Can you work these out from the model? Positions are in its coordinate system, mm. Face numbers are marked on the shaded views. A direction names the side the tool comes from. Coordinates: 2 decimals unless noted, no trailing zeros. Order: outer loops, then holes, each group sorted by start corner. A loop starts at its lowest first (then second) coordinate and runs counter-clockwise, first axis right, second up.
```python
from build123d import *

# Parameters (mm, degrees)
SKETCH1_W           = 3
SKETCH1_H           = 8.5
BOSS_EXTRUDE1_DEPTH = 0.25
SKETCH4_W           = 3
SKETCH4_H           = 0.5
CUT_EXTRUDE1_DEPTH  = 10.548715932
CHAMFER1_SIZE       = 0.7


with BuildPart() as part:
    # Sketch1 → Boss-Extrude1 (new body, symmetric)
    with BuildSketch(Plane(origin=(0, 0, 0), x_dir=(1, 0, 0), z_dir=(0, 1, 0))):
        Rectangle(SKETCH1_W, SKETCH1_H)
    extrude(amount=BOSS_EXTRUDE1_DEPTH, both=True)

    # Sweep1: sweep along a path in Sketch5
    with BuildLine(Plane(origin=(0, 0, 0), x_dir=(0, 0, -1), z_dir=(1, 0, 0))) as sweep1_path:
        Line((-6.415063509, -3.25), (-4.683012702, -0.25))
        ThreePointArc((-4.683012702, -0.25), (-4.5, -0.066987298), (-4.25, 0))
    # Sketch4 → Sweep1 (sweep)
    with BuildSketch(Plane.XY.offset(4.25)):
        Rectangle(SKETCH4_W, SKETCH4_H)
    sweep(path=sweep1_path.line)

    # Sketch6 → Cut-Extrude1 (cut, through all)
    with BuildSketch(Plane(origin=(0, 2.090303983, 3.620512702), x_dir=(1, 0, 0), z_dir=(0, 0.5, 0.866025404))):
        with BuildLine():
            Line((0.75, -2.472114317), (0.75, -3.972114317))
            ThreePointArc((0.75, -3.972114317), (0, -4.722114317), (-0.75, -3.972114317))
            Line((-0.75, -3.972114317), (-0.75, -2.472114317))
            ThreePointArc((-0.75, -2.472114317), (0, -1.722114317), (0.75, -2.472114317))
        make_face()
    extrude(amount=-CUT_EXTRUDE1_DEPTH, mode=Mode.SUBTRACT)

    # Chamfer1
    chamfer1_edges = [part.edges().sort_by_distance(p)[0] for p in [
        (-1.5, -3.25, 6.415063509),
        (1.5, -3.25, 6.415063509),
    ]]
    chamfer(chamfer1_edges, length=CHAMFER1_SIZE)


solid = part.part
```
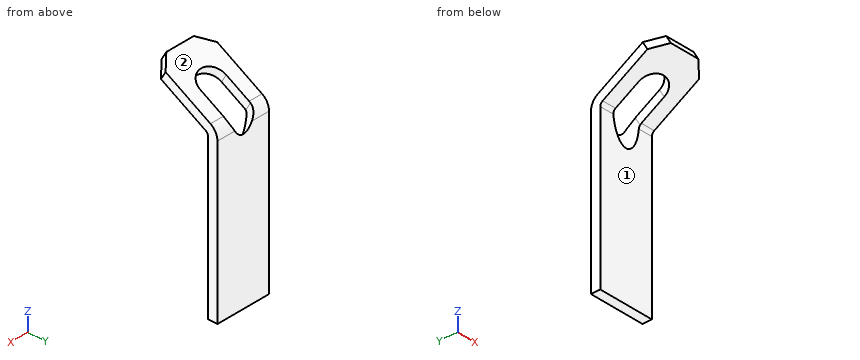
1. On a 3-axis mill with a long thin cutter (end or side, diameter ignored), from which of +Z, -Z, +X, -X, +Y, -Y can I reach the whole of each face in a straight line? I mean the marked faces 1 and 2. Say none if no direction works.
Completed:
face 1: -Z, +X, -X, -Y
face 2: +Z, +X, -X, +Y
2. Imagine slicing it at B-B on z = 5. Please give me the cut outline in (x, y), then the cut area to 3 significant figures.
Completed:
outline: (-1.5, -1.3) - (-0.75, -1.3) - (-0.75, -0.3) - (-1.5, -0.3) - close; (0.75, -1.3) - (1.5, -1.3) - (1.5, -0.3) - (0.75, -0.3) - close
area: 1.50 mm2
3. Imagine slicing it at D-D on z = -1. Please give me the cut outline in (x, y).
Completed:
outline: (-1.5, -0.25) - (1.5, -0.25) - (1.5, 0.25) - (-1.5, 0.25) - close
4. I'm going to push flat-ended pins straight in: pin 1 (1.5 mm diameter, centred on x = 0.5, z = 1.5, fed in from -Y); pin 2 (1.5 mm diameter, centred on x = -0.5, z = 4, fed in from -Y). Where does each tip first touch, or does it pass through?
Completed:
pin 1: stops at y = -0.25
pin 2: stops at y = -0.79
5. Please list where these lines run through material, in increasing order: probe 1 along Y at (x, z) = (-0.15, -3); probe 2 along Z at (x, y) = (-1.4, -0.6).
Completed:
probe 1: y = -0.25 to 0.25
probe 2: z = 4.6 to 5.17
6. Imagine slicing it at A-A on y = -0.85. Please give me the cut outline in (x, z).
Completed:
outline: (-1.5, 4.74) - (-0.75, 4.74) - (-0.75, 5.32) - (-1.5, 5.32) - close; (0.75, 4.74) - (1.5, 4.74) - (1.5, 5.32) - (0.75, 5.32) - close
